The listing builds one solid part. Answer for the finished solid, in the listing's coordinates (mm). A direction names the side the tool comes from. Round coordinates to 2 decimals unless told otherwise and drop trailing zeros. Loops run counter-clockwise (first coordinate to the right, second up) from the corner with the lowest first, then second, coordinate; pieces in that order, holes last. Notation, with made-up numbers: (65, -33) -> (109, -33) arc R25 cw to (109, 6) -> close; hole circle Ø6 at (39.25, 55.25). An arc over 180 degrees is marked (long way). Answer in a Markdown table with one row per item. Add a question column.
```python
from build123d import *

# Parameters (mm, degrees)
SKETCH010_R      = 0.95
EXTRUDE011_DEPTH = 10
EXTRUDE012_DEPTH = 50
SKETCH002_R      = 12.5
EXTRUDE002_DEPTH = 3
EXTRUDE001_DEPTH = 330
EXTRUDE013_DEPTH = 50


with BuildPart() as back_holes_e:
    # Sketch010 → Extrude011 (new body)
    with BuildSketch(Plane.XZ.offset(330)):
        with Locations((10.15, 89.481014)):
            Circle(SKETCH010_R)
        with Locations((72.35, 89.481014)):
            Circle(SKETCH010_R)
        with Locations((41.25, 10.15)):
            Circle(SKETCH010_R)
    extrude(amount=-EXTRUDE011_DEPTH)


with BuildPart() as drawer_back_support_negative_e:
    # Sketch014 (on Face14 of Extrude001) → Extrude012 (new body)
    with BuildSketch(Plane.XZ.offset(330)):
        Polygon((71.848171, 3.4), (79.1, 10.651829), (82.5, 10.651829), (82.5, 0), (0, 0), (0, 10.651829), (3.4, 10.651829), (10.651829, 3.4), align=None)
    extrude(amount=-EXTRUDE012_DEPTH)


with BuildPart() as drawer_back_support001:
    # Sweep: sweep along a path in Sketch012
    with BuildLine(Plane.XZ.offset(330)) as sweep_path:
        Line((15.9, 94.348171), (15.9, 15.9))
        Line((15.9, 15.9), (66.6, 15.9))
        Line((66.6, 15.9), (66.6, 94.348171))
    # Sketch009 (on Edge32 of Extrude001) → Sweep (sweep)
    with BuildSketch(Plane(origin=(52.866667, -110, 94.348171), x_dir=(-1, 0, 0), z_dir=(0, 0, -1))):
        Polygon((46.466667, -220), (36.966667, -220), (36.966667, -210), (46.466667, -200.5), align=None)
    sweep(path=sweep_path.line, is_frenet=True, transition=Transition.RIGHT)

    # Cut: cut drawer_back_support_negative_e
    add(drawer_back_support_negative_e.part, mode=Mode.SUBTRACT)

    # Cut002: cut back_holes_e
    add(back_holes_e.part, mode=Mode.SUBTRACT)


with BuildPart() as drawer_front_e:
    # Sketch002 (on Face13 of Extrude001) → Extrude002 (new body)
    with BuildSketch(Plane(origin=(0, 0, 0), x_dir=(-1, 0, 0), z_dir=(0, 1, 0))):
        Polygon((-82, 99.513856), (-79.5, 99.513856), (-72.013856, 107), (-72.013856, 109.5), (-10.486144, 109.5), (-10.486144, 107), (-3, 99.513856), (-0.5, 99.513856), (-0.5, 10.486144), (-3, 10.486144), (-10.086144, 3.4), (-10.651829, 3.4), (-71.848171, 3.4), (-72.413856, 3.4), (-79.5, 10.486144), (-82, 10.486144), align=None)
        with Locations((-41.25, 87.5)):
            Circle(SKETCH002_R, mode=Mode.SUBTRACT)
    extrude(amount=EXTRUDE002_DEPTH)


with BuildPart() as drawer_tube_e:
    # Sketch (on Face17 of Extrude) → Extrude001 (new body)
    with BuildSketch(Plane(origin=(0, 0, 0), x_dir=(-1, 0, 0), z_dir=(0, 1, 0))):
        Polygon((-79.1, 10.651829), (-71.848171, 3.4), (-10.651829, 3.4), (-3.4, 10.651829), (-3.4, 94.348171), (-6.4, 94.348171), (-6.4, 11.89447), (-11.89447, 6.4), (-70.60553, 6.4), (-76.1, 11.89447), (-76.1, 94.348171), (-79.1, 94.348171), align=None)
    extrude(amount=-EXTRUDE001_DEPTH)


with BuildPart() as drawer_front_support_negative_e:
    # Sketch015 (on Face13 of Extrude001) → Extrude013 (new body)
    with BuildSketch(Plane(origin=(0, 0, 0), x_dir=(-1, 0, 0), z_dir=(0, 1, 0))):
        Polygon((-3.4, 10.651829), (0, 10.651829), (0, 0), (-82.5, 0), (-82.5, 10.651829), (-79.1, 10.651829), (-71.848171, 3.4), (-10.651829, 3.4), align=None)
    extrude(amount=-EXTRUDE013_DEPTH)


with BuildPart() as drawer_inside:
    # Sweep001: sweep along a path in Sketch013
    with BuildLine(Plane.XZ) as sweep001_path:
        Line((16.4, 94.348171), (16.4, 16.4))
        Line((16.4, 16.4), (66.1, 16.4))
        Line((66.1, 16.4), (66.1, 94.348171))
    # Sketch011 (on Face6 of Extrude001) → Sweep001 (sweep)
    with BuildSketch(Plane.XY.offset(94.348171)):
        Polygon((6.4, 0), (6.4, -10), (16.4, 0), align=None)
    sweep(path=sweep001_path.line, is_frenet=True, transition=Transition.RIGHT)

    # Cut001: cut drawer_front_support_negative_e
    add(drawer_front_support_negative_e.part, mode=Mode.SUBTRACT)

    # Fusion: union drawer_back_support001, drawer_front_e, drawer_tube_e
    add(drawer_back_support001.part)
    add(drawer_front_e.part)
    add(drawer_tube_e.part)


solid = drawer_inside.part
```
Item 1: For faces 1 (the flat face through (7.077, -162.69, 6.975)), 2 (the flat face through (3.4, -163, 52)), 3 (the flat face through (15.9, -325, 55)), 4 (the flat face through (6.4, -158, 54)), determine the directions among +Z, -Z, +X, -X, +Y, -Y from which every point of the face is accessible in a straight line to the end or side of a thin tool.
Item 2: The mould has two halves that part along Y. Classify faces 5 (the flat face through (79.1, -163, 53)), 6 (the flat face through (67, -330, 39)), 7 (the flat face through (41, -158, 6.4)): +Y half, -Y half, draft (parallel to the pull), parting line (faces both ways), or undercut.
Item 3: Flat-ended cylindrical pins translate along their axes: P1, Ø0.6, axis at x = 10, z = 89.5, coming from the -Y side; P2, Ø8, axis at y = -323, z = 60, coming from the +X side; P3, Ø4, axis at y = -150, z = 19.5, coming from the -X side. Find the tip coordinate at first contact, or state that the pin passes through.
Item 4: Section A-A, the plane z = 81 is taken. Write down the section's boundary in (x, y).
Item 5: Section B-B, the plane y = -45 is taken. Write down the section's boundary in (x, z), and give its area (3 significant figures).
Item 6: Consider L1, parallel to X at y = -256, z = 15; L2, parallel to Y at x = 54.5, z = 71.5; L3, parallel to Z at x = 19, y = -92. Determine where each line is inside the solid, lowest interval first. Write a range as from..to.
Here are the results:
| question | item | result |
|---|---|---|
| 1 | face 1 | -Z, -X, -Y |
| 1 | face 2 | +Z, -Z, -X, -Y |
| 1 | face 3 | +Z, -Y |
| 1 | face 4 | +Z |
| 2 | face 5 | draft |
| 2 | face 6 | -Y half |
| 2 | face 7 | undercut |
| 3 | P1 | stops at y = -320 |
| 3 | P2 | stops at x = 79.1 |
| 3 | P3 | stops at x = 3.4 |
| 4 | outline | (0.5, 0) -> (3.4, 0) -> (3.4, -330) -> (15.9, -330) -> (15.9, -320) -> (6.4, -310.5) -> (6.4, -10) -> (16.4, 0) -> (30.57, 0) -> (30.57, 3) -> (0.5, 3) -> close; (51.93, 0) -> (66.1, 0) -> (76.1, -10) -> (76.1, -310.5) -> (66.6, -320) -> (66.6, -330) -> (79.1, -330) -> (79.1, 0) -> (82, 0) -> (82, 3) -> (51.93, 3) -> close |
| 5 | outline | (3.4, 10.65) -> (10.65, 3.4) -> (71.85, 3.4) -> (79.1, 10.65) -> (79.1, 94.35) -> (76.1, 94.35) -> (76.1, 11.89) -> (70.61, 6.4) -> (11.89, 6.4) -> (6.4, 11.89) -> (6.4, 94.35) -> (3.4, 94.35) -> close |
| 5 | area | 732 mm² |
| 6 | L1 | x = 3.4..6.4, 76.1..79.1 |
| 6 | L2 | y = 0..3 |
| 6 | L3 | z = 3.4..6.4 |
